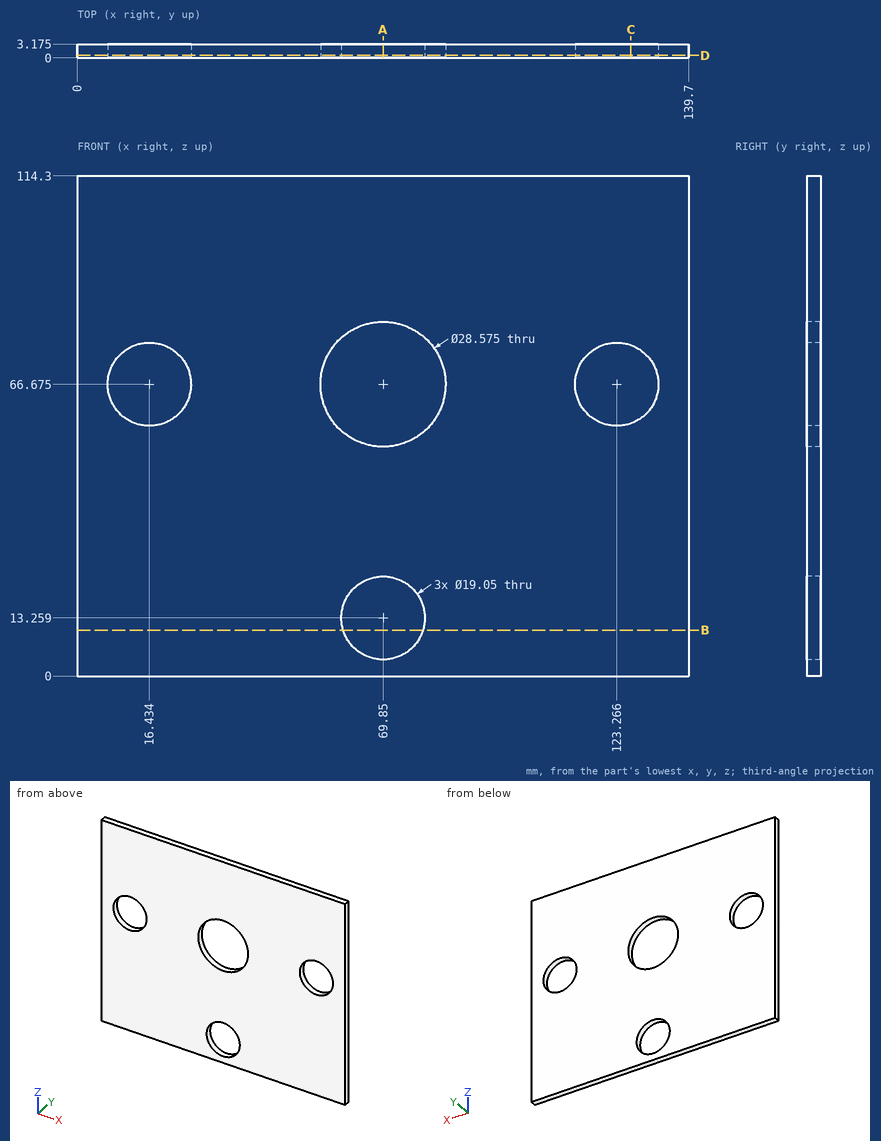
Design review of the part shown in the three views and the two pictorial views. Dimensions are in mm from the part's minimum x, y and z. Round coordinates to 2 decimals unless told otherwise and drop trailing zeros. Order: outer loops, then holes, each group sorted by start corner. A loop starts at its lowest first (then second) coordinate and runs counter-clockwise, first axis right, second up. Notation, with made-up numbers: (-23.75, 21) - (4.25, 21) arc R10 cw to (4.25, 27) - close; hole circle Ø6 at (-17, -28). An arc over 180 degrees is marked (long way). Answer in a Markdown table with one row per item.
(1) For line 1 (X direction, y = 1.9, z = 62) (1 decimal); line 2 (X direction, y = 2.15, z = 58) (1 decimal); line 3 (Z direction, x = 75, y = 0.75), list the stretches that pass through material, from the lowest coordinate up. Write a range as from..to.
Result set:
| item | result |
|---|---|
| line 1 | x = 0..8.1, 24.7..56.3, 83.4..115, 131.6..139.7 |
| line 2 | x = 0..12.5, 20.4..58.5, 81.2..119.3, 127.2..139.7 |
| line 3 | z = 0..5.25, 21.27..53.35, 80..114.3 |
(2) Clearance check with a flat-ended pin moving along its axis: P1, Ø17, axis at x = 69.85, z = 13.26, coming from the -Y side (1 decimal). State where the tip first meets the part, or that it passes through.
Result set:
| item | result |
|---|---|
| P1 | passes through |
(3) Take a section at A-A on x = 69.85. Write out the cut boundary in (y, z) (1 decimal), plus the area to 3 significant figures.
Result set:
| item | result |
|---|---|
| outline | (0, 0) - (3.2, 0) - (3.2, 3.7) - (0, 3.7) - close; (0, 22.8) - (3.2, 22.8) - (3.2, 52.4) - (0, 52.4) - close; (0, 81) - (3.2, 81) - (3.2, 114.3) - (0, 114.3) - close |
| area | 212 mm2 |
(4) Take a section at B-B on z = 10.5. Write out the cut boundary in (x, y) (1 decimal).
Result set:
| item | result |
|---|---|
| outline | (0, 0) - (60.7, 0) - (60.7, 3.2) - (0, 3.2) - close; (79, 0) - (139.7, 0) - (139.7, 3.2) - (79, 3.2) - close |
(5) Take a section at C-C on x = 126.5. Write out the cut boundary in (y, z) (1 decimal), plus the area to 3 significant figures.
Result set:
| item | result |
|---|---|
| outline | (0, 0) - (3.2, 0) - (3.2, 57.7) - (0, 57.7) - close; (0, 75.6) - (3.2, 75.6) - (3.2, 114.3) - (0, 114.3) - close |
| area | 306 mm2 |
(6) Take a section at D-D on y = 0.55. Count the separate pieces of the cut face and the enclosed holes in it, plus the area to 3 significant figures.
Result set:
| item | result |
|---|---|
| separate pieces | 1 |
| enclosed holes | 4 |
| area | 14,500 mm2 |
